Study the drawing (mm; zero at the part's minimum x, y, z) and answer. A direction names the side the tool comes from. Round coordinates to 2 decimals unless told otherwise and drop trailing zeros. Loops run counter-clockwise (first coordinate to the right, second up) from the corner with the lowest first, then second, coordinate; pieces in that order, holes last. Notation, with made-up numbers: (54.5, -34) -> (110.5, -34) arc R23 cw to (110.5, -10) -> close; hole circle Ø5 at (73.5, -31.5). An arc over 180 degrees is marked (long way). Write each question's results on one line, items separated by ' | '. Start each with the question number.
(1) The part is cut by section D-D (x = 5). Determine the outline of the cut face in (y, z).
(2) Flat-ended cylindrical pins translate along their axes: pin 1 (23.5 mm diameter, centred on x = 46.5, z = 58, fed in from -Y); pin 2 (8.5 mm diameter, centred on x = 44, z = 41, fed in from +Y); pin 3 (23.5 mm diameter, centred on x = 39.1, z = 39.26, fed in from +Y); pin 4 (5 mm diameter, centred on x = 71.5, z = 63.5, fed in from -Y). Find the tip coordinate at first contact, or state that the pin passes through.
(3) The part is cut by section B-B (z = 30). Determine the outline of the cut face in (x, y), plus the area to 3 significant figures.
(4) For the marked faces 5 and 6, determine the directions among +Z, -Z, +X, -X, +Y, -Y from which every point of the face is accessible in a straight line to the end or side of a thin tool.
(5) Straight lines are drawn through the part: probe 1 along Y at (x, z) = (60, 15); probe 2 along X at (y, z) = (66.5, 45.5); probe 3 along Z at (x, y) = (38, 32). For each, find the intervals that lie inside material, in ascending order.
(6) The part is cut by section A-A (x = 35). Determine the outline of the cut face in (y, z) (1 decimal), plus the area to 3 significant figures.
(7) The part is cut by section C-C (y = 52). Determine the outline of the cut face in (x, z), plus the area to 3 significant figures.
(8) Determine the mould class of the marked faces 1, 2, 3 and 4 for opening direction Z: released by +Z, released by -Z, zero draft, split by the parting line, or undercut.
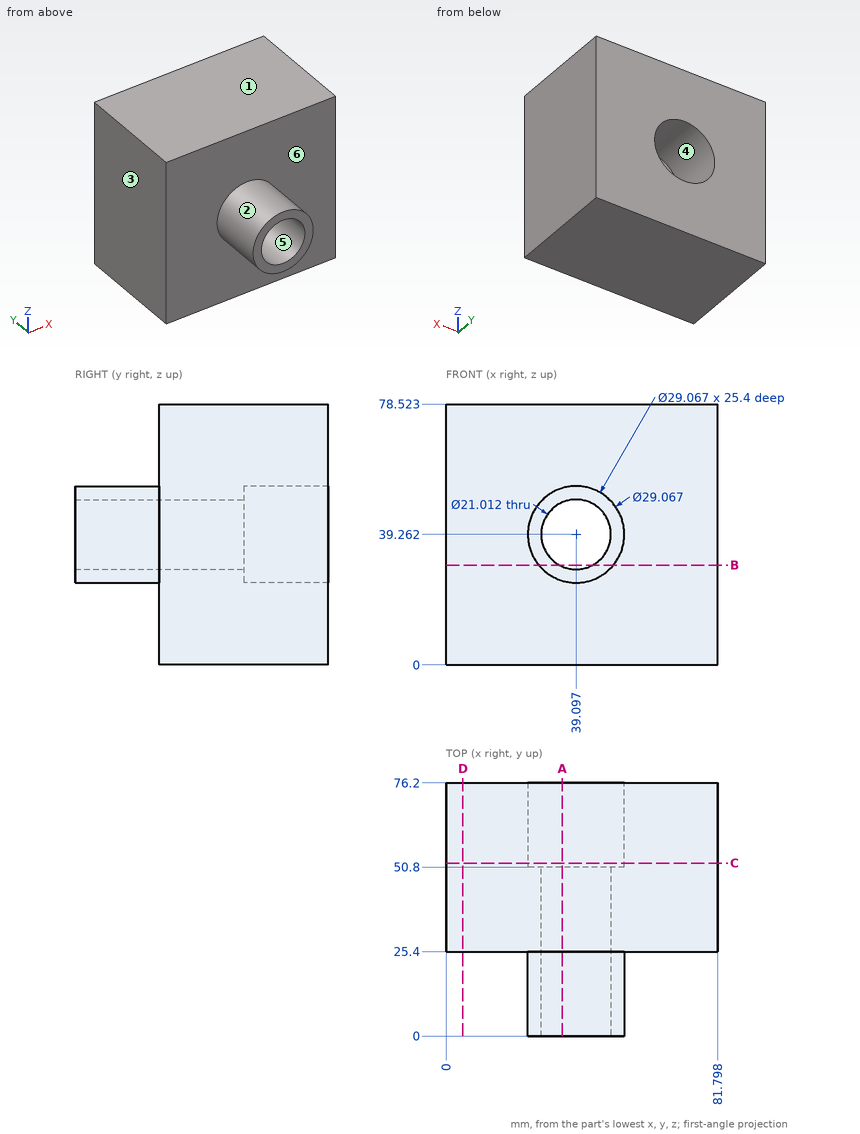
Checked values:
1) outline: (25.4, 0) -> (76.2, 0) -> (76.2, 78.52) -> (25.4, 78.52) -> close
2) pin 1: stops at y = 0 | pin 2: passes through | pin 3: stops at y = 50.8 | pin 4: stops at y = 25.4
3) outline: (0, 25.4) -> (27.9, 25.4) -> (27.9, 0) -> (34.14, 0) -> (34.14, 50.8) -> (27.9, 50.8) -> (27.9, 76.2) -> (0, 76.2) -> close; (44.06, 0) -> (50.3, 0) -> (50.3, 25.4) -> (81.8, 25.4) -> (81.8, 76.2) -> (50.3, 76.2) -> (50.3, 50.8) -> (44.06, 50.8) -> close | area: 3,650 mm2
4) face 5: +Y, -Y | face 6: -Y
5) probe 1: y = 25.4 to 76.2 | probe 2: x = 0 to 25.97, 52.22 to 81.8 | probe 3: z = 0 to 28.81, 49.71 to 78.52
6) outline: (0, 25.3) -> (25.4, 25.3) -> (25.4, 0) -> (76.2, 0) -> (76.2, 25.3) -> (50.8, 25.3) -> (50.8, 29.6) -> (0, 29.6) -> close; (0, 48.9) -> (50.8, 48.9) -> (50.8, 53.2) -> (76.2, 53.2) -> (76.2, 78.5) -> (25.4, 78.5) -> (25.4, 53.2) -> (0, 53.2) -> close | area: 3,010 mm2
7) outline: (0, 0) -> (81.8, 0) -> (81.8, 78.52) -> (0, 78.52) -> close; hole circle Ø29.07 at (39.1, 39.26) | area: 5,760 mm2
8) face 1: released by +Z | face 2: split by the parting line | face 3: zero draft | face 4: undercut
